```python
from build123d import *

# Parameters (mm, degrees)
SKETCH1_W           = 80
SKETCH1_H           = 80
SKETCH1_R           = 15
SKETCH1_W_2         = 30
SKETCH1_H_2         = 30
BOSS_EXTRUDE1_DEPTH = 10


with BuildPart() as part:
    # Sketch1 → Boss-Extrude1 (new body)
    with BuildSketch(Plane.XY):
        Rectangle(SKETCH1_W, SKETCH1_H)
        with Locations((-20, 20)):
            Circle(SKETCH1_R, mode=Mode.SUBTRACT)
        Polygon((11.339745962, 35), (2.679491924, 20), (11.339745962, 5), (28.660254038, 5), (37.320508076, 20), (28.660254038, 35), align=None, mode=Mode.SUBTRACT)
        with Locations((0, -22)):
            Rectangle(SKETCH1_W_2, SKETCH1_H_2, mode=Mode.SUBTRACT)
    extrude(amount=-BOSS_EXTRUDE1_DEPTH)


solid = part.part
```
Here's how the part is built. I have some questions about the finished solid (model axes, mm). A direction names the side the tool comes from. Coordinates: 2 decimals unless noted, no trailing zeros. Order: outer loops, then holes, each group sorted by start corner. A loop starts at its lowest first (then second) coordinate and runs counter-clockwise, first axis right, second up.
1) I need wall thicknesses on line 1 (Y direction, x = -20, z = -7.5); line 2 (X direction, y = -36, z = -1.75); line 3 (Y direction, x = 14.5, z = -8). Which ranges of each line are inside material? Lowest first, please.
2) Imagine slicing it at C-C on z = -7.5. List the corners of the cut face in (x, y) for me, and give its area (3 significant figures).
3) Will this pin go through, and if not, where does the flat tip stop? pin 1 (1 mm diameter, centred on x = 21, y = -23.5, fed in from +Z).
4) Which directions (+Z, -Z, +X, -X, +Y, -Y) give clear straight access to the entire face, cutting with the end or side of a thin tool? Please do faces 5 (the face through (33.05, 27.4, -4.93)), 6 (the face through (-1, -40, -5)).
5) Imagine slicing it at A-A on x = -32. List the corners of the cut face in (y, z) for me, and give its area (3 significant figures).
6) Imagine slicing it at B-B on y = -20.5. List the corners of the cut face in (x, z) for me, and give its area (3 significant figures).
7) We'd pull the mould along X, two halves only. Please class faces 1 (the face through (0, -7, -5)), 2 (the face through (40, -1, -5)), 3 (the face through (7.07, 27.605, -4.93)), 4 (the face through (-1, 1, -10)): +X half, -X half, draft (parallel to the pull), parting line (faces both ways), or undercut.
8) Imagine slicing it at D-D on x = -9.5. List the corners of the cut face in (y, z) for me, and give its area (3 significant figures).
Response values:
1. line 1: y = -40 to 5, 35 to 40
1. line 2: x = -40 to -15, 15 to 40
1. line 3: y = -40 to -37, -7 to 5, 35 to 40
2. outline: (-40, -40) - (40, -40) - (40, 40) - (-40, 40) - close; hole circle Ø30 at (-20, 20); hole (-15, -37) - (15, -37) - (15, -7) - (-15, -7) - close; hole (2.68, 20) - (11.34, 5) - (28.66, 5) - (37.32, 20) - (28.66, 35) - (11.34, 35) - close
2. area: 4,010 mm2
3. pin 1: stops at z = 0
4. face 5: +Z, -Z
4. face 6: +Z, -Z, +X, -X, -Y
5. outline: (-40, -10) - (11, -10) - (11, 0) - (-40, 0) - close; (29, -10) - (40, -10) - (40, 0) - (29, 0) - close
5. area: 620 mm2
6. outline: (-40, -10) - (-15, -10) - (-15, 0) - (-40, 0) - close; (15, -10) - (40, -10) - (40, 0) - (15, 0) - close
6. area: 500 mm2
7. face 1: undercut
7. face 2: +X half
7. face 3: undercut
7. face 4: draft
8. outline: (-40, -10) - (-37, -10) - (-37, 0) - (-40, 0) - close; (-7, -10) - (9.29, -10) - (9.29, 0) - (-7, 0) - close; (30.71, -10) - (40, -10) - (40, 0) - (30.71, 0) - close
8. area: 286 mm2
